Verification items for this drawing (mm, ordinates from the low corner). A direction names the side the tool comes from. Round coordinates to 2 decimals unless told otherwise and drop trailing zeros. Write each loop counter-clockwise with the first axis right and the second up, starting at its lowest first coordinate (ties: lowest second). Pieces come first, ordered by that corner, then holes. Notation, with made-up numbers: M -10.75,19.5 L 39.25,19.5 A8 cw 39.25,34.5 Z; hole C 89.5,7.25 d8. An arc over 180 degrees is marked long. One line per question, with ' | ' between items. Start each with the question number.
Q1. Tool access check on the marked faces 1 and 2. Record the directions out of +Z, -Z, +X, -X, +Y, -Y that give a thin tool (end or side, any length) a straight path to the whole face; none if there is none.
Q2. Cross-section at C-C (x = 4). Record the boundary of the cut face in (y, z).
Q3. Cross-section at B-B (y = 26). Record the boundary of the cut face in (x, z).
Q4. Release check for a two-part mould opening along X. For the marked faces 3, 4 and 5 record: released by +X, released by -X, zero draft, split by the parting line, or undercut.
Q5. Cross-section at A-A (z = 4). Record the boundary of the cut face in (x, y), then the cut area to 3 significant figures.
Q6. Gauge pin test, flat end, axial feed: pin 1 (1 mm diameter, centred on x = 2, y = 9.5, fed in from +Z). Record the tip position at first contact, or that the pin passes through.
Q7. Thickness scan on line 1 along Y through (x, z) = (1.5, 2); line 2 along X through (y, z) = (26.75, 4); line 3 along X through (y, z) = (21.5, 3.5). Record the ranges inside material, lowest first. Write a range as from..to.
Q8. Cross-section at D-D (y = 6.75). Record the boundary of the cut face in (x, z).
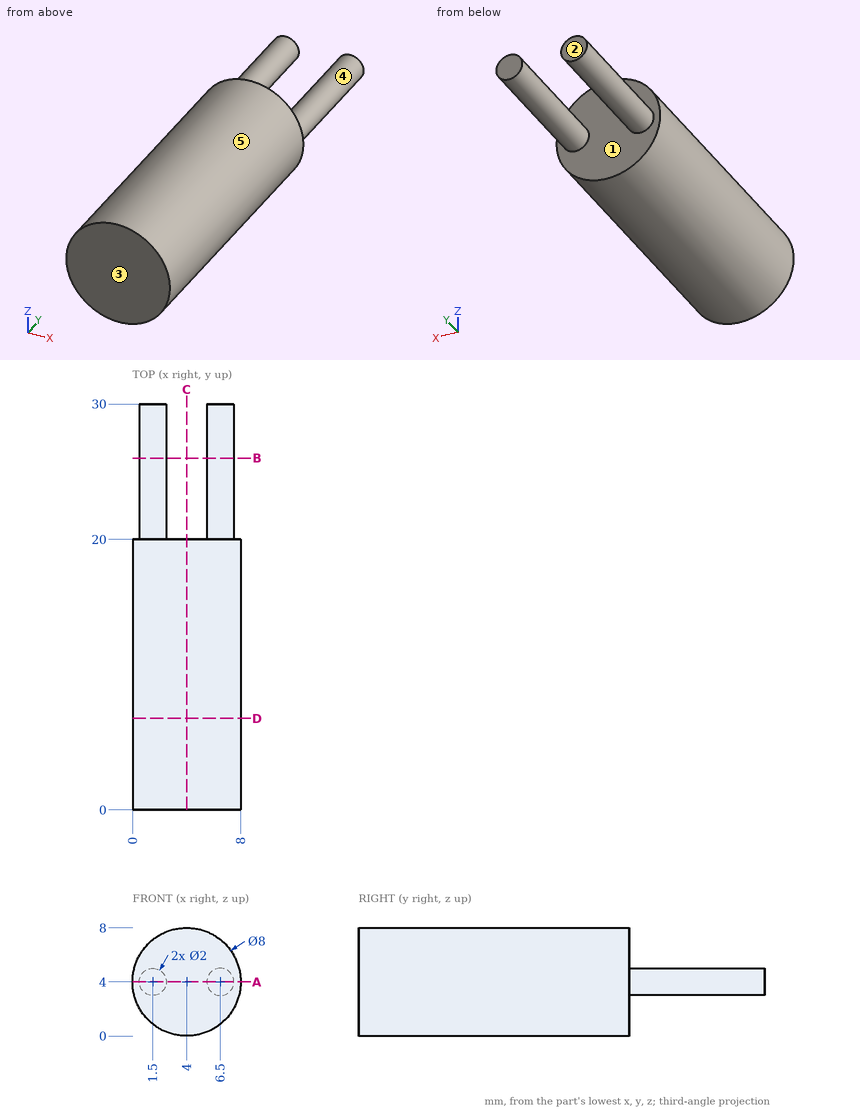
Determined:
1) face 1: +Y | face 2: +Z, -Z, +X, -X, +Y
2) outline: M 0,0 L 20,0 L 20,8 L 0,8 Z
3) outline: C 1.5,4 d2; C 6.5,4 d2
4) face 3: zero draft | face 4: undercut | face 5: split by the parting line
5) outline: M 0,0 L 8,0 L 8,20 L 7.5,20 L 7.5,30 L 5.5,30 L 5.5,20 L 2.5,20 L 2.5,30 L 0.5,30 L 0.5,20 L 0,20 Z | area: 200 mm²
6) pin 1: stops at z = 7.71
7) line 1: y = 0..20 | line 2: x = 0.5..2.5, 5.5..7.5 | line 3: x = 0.63..2.37, 5.63..7.37
8) outline: C 4,4 d8
